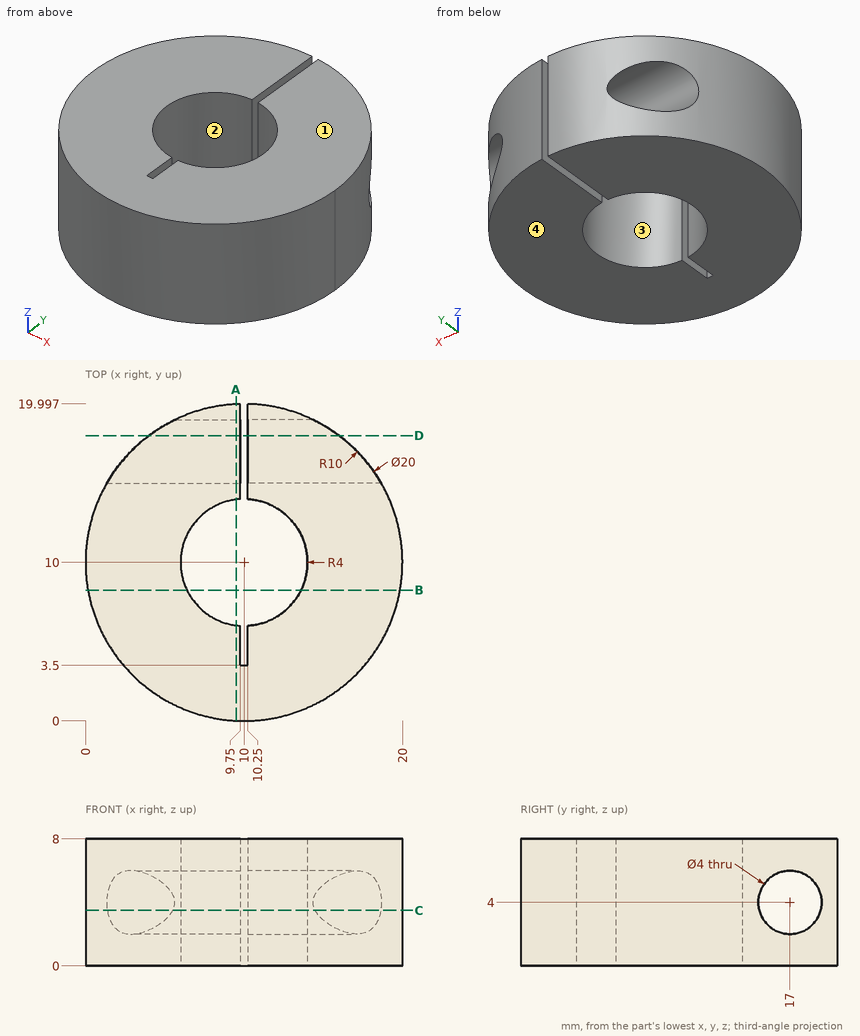
Verification items for this drawing (mm, ordinates from the low corner). A direction names the side the tool comes from. Give positions to 0.01 mm unless a question says otherwise; leave off trailing zeros. Loops run counter-clockwise (first coordinate to the right, second up) from the corner with the lowest first, then second, coordinate; pieces in that order, holes last.
1. Cross-section at D-D on y = 18. Record the cut outline in (x, z).
Derived:
outline: (4, 0) - (9.75, 0) - (9.75, 2.27) - (4, 2.27) - close; (4, 5.73) - (9.75, 5.73) - (9.75, 8) - (4, 8) - close; (10.25, 0) - (16, 0) - (16, 2.27) - (10.25, 2.27) - close; (10.25, 5.73) - (16, 5.73) - (16, 8) - (10.25, 8) - close
2. Cross-section at C-C on z = 3.5. Record the cut outline in (x, y).
Derived:
outline: (1.38, 15.06) arc R10 ccw (long way) to (18.62, 15.06) - (10.25, 15.06) - (10.25, 13.99) arc R4 cw to (10.25, 6.01) - (10.25, 3.5) - (9.75, 3.5) - (9.75, 6.01) arc R4 cw to (9.75, 13.99) - (9.75, 15.06) - close; (5.51, 18.94) - (9.75, 18.94) - (9.75, 20) arc R10 ccw to start; (10.25, 18.94) - (14.49, 18.94) arc R10 ccw to (10.25, 20) - close
3. Cross-section at B-B on y = 8.25. Record the cut outline in (x, z).
Derived:
outline: (0.15, 0) - (6.4, 0) - (6.4, 8) - (0.15, 8) - close; (13.6, 0) - (19.85, 0) - (19.85, 8) - (13.6, 8) - close
4. Material ranges on probe 1 along X at (y, z) = (15, 6.75); probe 2 along Y at (x, z) = (12, 5.75) (1 decimal); probe 3 along Y at (x, z) = (7, 4) (1 decimal), recorded low to high.
Derived:
probe 1: x = 1.34 to 9.75, 10.25 to 18.66
probe 2: y = 0.2 to 6.5, 13.5 to 16, 18 to 19.8
probe 3: y = 0.5 to 7.4, 12.6 to 15, 19 to 19.5
5. Release check for a two-part mould opening along Y. For the marked faces 1 and 2 record: +Y half, -Y half, draft (parallel to the pull), parting line (faces both ways), or undercut.
Derived:
face 1: draft
face 2: undercut
6. Cross-section at A-A on x = 9.5. Record the cut outline in (y, z).
Derived:
outline: (0.01, 0) - (6.03, 0) - (6.03, 8) - (0.01, 8) - close; (13.97, 0) - (19.99, 0) - (19.99, 8) - (13.97, 8) - close; hole circle Ø4 at (17, 4)
7. Go/stop test with flat-tipped pins: P1, Ø2, axis at x = 4, z = 5.5, coming from the +Y side; P2, Ø2, axis at y = 5, z = 3.5, coming from the +X side (3 decimals); P3, Ø4, axis at y = 2, z = 7, coming from the -X side. Record where each tip stops, or that it passes through.
Derived:
P1: stops at y = 18.66
P2: stops at x = 19.165
P3: stops at x = 2
8. Tool access check on the marked faces 3 and 4. Record the directions out of +Z, -Z, +X, -X, +Y, -Y that give a thin tool (end or side, any length) a straight path to the whole face; none if there is none.
Derived:
face 3: +Z, -Z
face 4: -Z, +X, -X, +Y, -Y
